Design review of the part built by this model. Coordinates are the model's own, in mm. A direction names the side the tool comes from. Coordinates: 2 decimals unless noted, no trailing zeros. Loops run counter-clockwise (first coordinate to the right, second up) from the corner with the lowest first, then second, coordinate; pieces in that order, holes last. Notation, with made-up numbers: (14, 84) - (26, 84) arc R21 ccw to (26, 99) - close; hole circle Ø2 at (32, 18). An arc over 180 degrees is marked (long way). Answer in a Markdown table with one row per item. Add a question column.
(1) Clearance check with flat-ended pins moving along their axes: pin 1 (1.5 mm diameter, centred on y = 6, z = 1, fed in from +X); pin 2 (1.5 mm diameter, centred on x = 13, z = 1.5, fed in from -Y). State where each tip first meets the part, or that it passes through.
(2) We need section C-C, the plane x = -17.5. Write out the cut boundary in (y, z).
(3) The part is to be moulded in two halves that separate along Y. For faces 1 (the face through (0.93, 7.09, 1.82)), 2 (the face through (1.02, 7.76, -0.61)), 3 (the face through (-1, 49.5, 2)), 4 (the face through (50.72, -50.49, -0.51)), say which applies: released by +Y, released by -Y, zero draft, split by the parting line, or undercut.
(4) To check wall thickness, follow L1, parallel to Y at x = 0, z = -0.7 (3 decimals); L2, parallel to Y at x = 0, z = 0.95; L3, parallel to X at y = 27, z = 3.1. State the ranges of each line that lie inside material, in increasing order. Write a range as [from, to].
(5) We need section A-A, the plane x = 0. Write out the cut boundary in (y, z) (3 decimals).
(6) We need section D-D, the plane z = 2.25. Write out the cut boundary in (x, y).
(7) For faces 5 (the face through (49.5, -1, 2)), 6 (the face through (-49.5, -1, 2)), 7 (the face through (-1, -49.5, 2)), list the 3-axis set-ups (+Z, -Z, +X, -X, +Y, -Y) from which the entire face can be reached by the end or side of a thin tool; tool diameter is ignored.
from build123d import *

# Parameters (mm, degrees)
SKETCH_1_W          = 99
SKETCH_1_H          = 99
EXTRUDE_1_DEPTH     = 3.9
SKETCH_2_W          = 110
SKETCH_2_H          = 110
EXTRUDE_2_DEPTH     = 1
SKETCH_3_R          = 7.15
CUT_EXTRUDE_1_DEPTH = 78.935935229
SKETCH_5_R          = 7.825
CUT_EXTRUDE_2_DEPTH = 0.8
FILLET_1_R          = 15


with BuildPart() as part:
    # 草图1 → 凸台-拉伸1 (new body)
    with BuildSketch(Plane.XY):
        Rectangle(SKETCH_1_W, SKETCH_1_H)
    extrude(amount=EXTRUDE_1_DEPTH)

    # 草图2 → 凸台-拉伸2 (add)
    with BuildSketch(Plane(origin=(0, 0, 0), x_dir=(-1, 0, 0), z_dir=(0, 0, -1))):
        Rectangle(SKETCH_2_W, SKETCH_2_H)
    extrude(amount=EXTRUDE_2_DEPTH)

    # 草图3 → 切除-拉伸1 (cut, through all)
    with BuildSketch(Plane(origin=(0, 0, -1), x_dir=(-1, 0, 0), z_dir=(0, 0, -1))):
        Circle(SKETCH_3_R)
    extrude(amount=-CUT_EXTRUDE_1_DEPTH, mode=Mode.SUBTRACT)

    # 草图5 → 切除-拉伸2 (cut)
    with BuildSketch(Plane(origin=(0, 0, -1), x_dir=(-1, 0, 0), z_dir=(0, 0, -1))):
        Circle(SKETCH_5_R)
    extrude(amount=-CUT_EXTRUDE_2_DEPTH, mode=Mode.SUBTRACT)

    # 圆角1
    fillet_1_edges = [part.edges().sort_by_distance(p)[0] for p in [
        (-55, -55, -0.5),
        (-55, 55, -0.5),
        (55, 55, -0.5),
        (55, -55, -0.5),
    ]]
    fillet(fillet_1_edges, radius=FILLET_1_R)


solid = part.part
Responses:
| question | item | result |
|---|---|---|
| 1 | pin 1 | stops at x = 49.5 |
| 1 | pin 2 | stops at y = -49.5 |
| 2 | outline | (-55, -1) - (55, -1) - (55, 0) - (49.5, 0) - (49.5, 3.9) - (-49.5, 3.9) - (-49.5, 0) - (-55, 0) - close |
| 3 | face 1 | undercut |
| 3 | face 2 | undercut |
| 3 | face 3 | released by +Y |
| 3 | face 4 | released by -Y |
| 4 | L1 | y = [-55, -7.825], [7.825, 55] |
| 4 | L2 | y = [-49.5, -7.15], [7.15, 49.5] |
| 4 | L3 | x = [-49.5, 49.5] |
| 5 | outline | (-55, -1) - (-7.825, -1) - (-7.825, -0.2) - (-7.15, -0.2) - (-7.15, 3.9) - (-49.5, 3.9) - (-49.5, 0) - (-55, 0) - close; (7.15, -0.2) - (7.825, -0.2) - (7.825, -1) - (55, -1) - (55, 0) - (49.5, 0) - (49.5, 3.9) - (7.15, 3.9) - close |
| 6 | outline | (-49.5, -49.5) - (49.5, -49.5) - (49.5, 49.5) - (-49.5, 49.5) - close; hole circle Ø14.3 at (0, 0) |
| 7 | face 5 | +Z, +X, +Y, -Y |
| 7 | face 6 | +Z, -X, +Y, -Y |
| 7 | face 7 | +Z, +X, -X, -Y |
